Read the model definition and answer for the solid it produces. Units are mm, in the model's axes. A direction names the side the tool comes from. Give positions to 0.01 mm unless a question says otherwise; leave off trailing zeros. Answer as CSV lines item,"result". Start each with the question number.
from build123d import *

# Parameters (mm, degrees)
F2_W     = 6.985
F2_H     = 6.985
F3_DEPTH = 31.3591392294
F4_R     = 1.27
F5_DEPTH = 31.3591393294


with BuildPart() as f1:
    # F0 (on Right) → F1 (revolve)
    with BuildSketch(Plane.YZ):
        with BuildLine():
            Line((0, 0), (0, 31.3581392294))
            Line((0, 31.3581392294), (-38.1, 31.3581392294))
            Line((-38.1, 31.3581392294), (-38.1, 29.0615208854))
            add(Edge.make_bspline(
                [(-38.1, 29.0615208854), (-26.7971571911, 25.1598302044), (-15.8579765578, 15.5865226046), (-12.8539522067, 8.1840861578), (-12.014542318, 0)],
                knots=[0.1026687543, 0.1026687543, 0.1026687543, 0.1026687543, 0.586312354, 1, 1, 1, 1], degree=3))
            Line((-12.014542318, 0), (0, 0))
        make_face()
    revolve(axis=Axis((0, 0, 15.6790696147), (0, 0, -1)))

    # F2 (on Top) → F3 (cut, through all)
    with BuildSketch(Plane.XY):
        Rectangle(F2_W, F2_H)
    extrude(amount=F3_DEPTH, mode=Mode.SUBTRACT)

    # F4 (on face) → F5 (cut, through all)
    with BuildSketch(Plane.XY.offset(31.3581392294)):
        with Locations((-25.4, 0)):
            Circle(F4_R)
        with Locations((25.4, 0)):
            Circle(F4_R)
    extrude(amount=-F5_DEPTH, mode=Mode.SUBTRACT)


solid = f1.part
(1) Determine the mould class of faces 3 (the cylindrical face through (23.183, 30.235, 30.194)), 4 (the flat face through (0, -3.492, 15)), 5 (the flat face through (-1, 8, 31.358)), 6 (the cylindrical face through (24.13, 0.06, 26.75)) for opening direction X: released by +X, released by -X, zero draft, split by the parting line, or undercut.
(2) Flat-ended cylindrical pins translate along their axes: pin 1 Ø2 at (y, z) = (-7.5, 22) entering from -X; pin 2 Ø1.5 at (y, z) = (-12.5, 19.5) entering from -X; pin 3 Ø3.5 at (x, z) = (-0.5, 20.5) entering from -Y; pin 4 Ø4 at (x, y) = (25.4, 0) entering from +Z. Find the tip coordinate at first contact, or state that the pin passes through.
(3) Straight lines are drawn through the part: line 1 (X direction, y = 0, z = 29.25); line 2 (X direction, y = 0, z = 27.25); line 3 (X direction, y = 1, z = 21.5). For each, find the intervals that lie inside material, in ascending order. Write a range as [from, to].
(4) Section A-A, the plane y = 0 is taken. State how many separate pieces and enclosed holes the cut face has, and give its area (3 significant figures).
(5) Which of the six approach directions +Z, -Z, +X, -X, +Y, -Y give full straight-line access (tool end or side, diameter ignored) to faces 1 (the flat face through (0, -5, 0)), 2 (the flat face through (0, 3.492, 15))?
Checks:
1,face 3,"split by the parting line"
1,face 4,"undercut"
1,face 5,"zero draft"
1,face 6,"undercut"
2,pin 1,"stops at x = -24.44"
2,pin 2,"stops at x = -18.11"
2,pin 3,"stops at y = -24.45"
2,pin 4,"stops at z = 31.36"
3,line 1,"x = [-38.1, -26.67], [-24.13, -3.49], [3.49, 24.13], [26.67, 38.1]"
3,line 2,"x = [-33.42, -26.67], [-24.13, -3.49], [3.49, 24.13], [26.67, 33.42]"
3,line 3,"x = [-23.43, -3.49], [3.49, 23.43]"
4,separate pieces,"4"
4,enclosed holes,"0"
4,area,"1,030 mm²"
5,face 1,"-Z, +X, -X, +Y, -Y"
5,face 2,"+Z, -Z"
